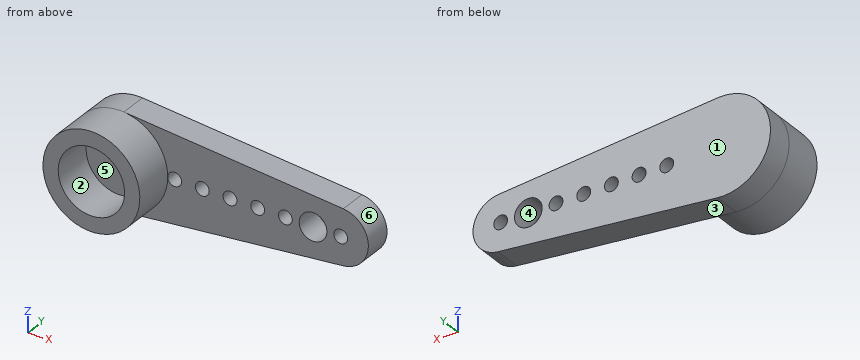
from build123d import *

# Parameters (mm, degrees)
SKETCH1_R           = 3.5
SKETCH1_R_2         = 2.4
BOSS_EXTRUDE1_DEPTH = 3
SKETCH2_R           = 1
SKETCH2_R_2         = 0.5
BOSS_EXTRUDE2_DEPTH = 2


with BuildPart() as part:
    # Sketch1 → Boss-Extrude1 (new body)
    with BuildSketch(Plane(origin=(0, 0, 0), x_dir=(1, 0, 0), z_dir=(0, 1, 0))):
        with Locations(Location((0, 0, 0), (0, 0, 270))):
            Circle(SKETCH1_R)
        with Locations(Location((0, 0, 0), (0, 0, 270))):
            Circle(SKETCH1_R_2, mode=Mode.SUBTRACT)
    extrude(amount=BOSS_EXTRUDE1_DEPTH)

    # Sketch2 → Boss-Extrude2 (add)
    with BuildSketch(Plane(origin=(0, 3, 0), x_dir=(1, 0, 0), z_dir=(0, 1, 0))):
        with BuildLine():
            Line((16.1875, 1.99119154), (0.328125, 3.484585195))
            ThreePointArc((0.328125, 3.484585195), (-3.5, 0), (0.328125, -3.484585195))
            Line((0.328125, -3.484585195), (16.1875, -1.99119154))
            ThreePointArc((16.1875, -1.99119154), (18, 0), (16.1875, 1.99119154))
        make_face()
        with Locations(Location((14, 0, 0), (0, 0, 270))):
            Circle(SKETCH2_R, mode=Mode.SUBTRACT)
        with Locations(Location((4, 0, 0), (0, 0, 180))):
            Circle(SKETCH2_R_2, mode=Mode.SUBTRACT)
        with Locations(Location((6, 0, 0), (0, 0, 270))):
            Circle(SKETCH2_R_2, mode=Mode.SUBTRACT)
        with Locations(Location((8, 0, 0), (0, 0, 270))):
            Circle(SKETCH2_R_2, mode=Mode.SUBTRACT)
        with Locations(Location((10, 0, 0), (0, 0, 270))):
            Circle(SKETCH2_R_2, mode=Mode.SUBTRACT)
        with Locations(Location((12, 0, 0), (0, 0, 270))):
            Circle(SKETCH2_R_2, mode=Mode.SUBTRACT)
        with Locations(Location((16, 0, 0), (0, 0, 270))):
            Circle(SKETCH2_R_2, mode=Mode.SUBTRACT)
    extrude(amount=BOSS_EXTRUDE2_DEPTH)


solid = part.part
Input: part model. Units: mm. Frame: model coordinates. Face numbers are marked on the shaded views. A direction names the side the tool comes from. Coordinates: 2 decimals unless noted, no trailing zeros. Loops run counter-clockwise (first coordinate to the right, second up) from the corner with the lowest first, then second, coordinate; pieces in that order, holes last.
Q1. Cut plane B-B (y = 3.65). Output: boundary loops of the cut face in (x, z).
Q2. Set-up query: the marked faces 5 and 6. Return all of +Z, -Z, +X, -X, +Y, -Y with unobstructed straight access to the full face (end or side cutting, diameter ignored); none if empty.
Q3. Cut plane A-A (x = 4). Output: boundary loops of the cut face in (y, z), then the cut area to 3 significant figures.
Q4. Material intervals for line 1 (X direction, y = 1.65, z = 0); line 2 (X direction, y = 1.9, z = -2); line 3 (Y direction, x = -1.5, z = 1), sorted ascending.
Q5. Cut plane C-C (x = 0). Output: boundary loops of the cut face in (y, z).
Q6. Draft query along Z for the marked faces 1, 2, 3 and 4. Return one class per face: +Z half, -Z half, draft (parallel to the pull), parting line (faces both ways), or undercut.
Q7. Cut plane D-D (y = 0.6). Output: boundary loops of the cut face in (x, z).
Q8. Contact query for flat-ended pins moving along their axis: pin 1 (1.8 mm diameter, centred on x = 14, z = 0, fed in from -Y); pin 2 (3 mm diameter, centred on y = 3, z = -2.5, fed in from +X); pin 3 (4 mm diameter, centred on x = 7.5, z = -2.5, fed in from -Y). Output: stop coordinate, or through.
Working result:
1. outline: (0.33, -3.48) - (16.19, -1.99) arc R2 ccw to (16.19, 1.99) - (0.33, 3.48) arc R3.5 ccw (long way) to start; hole circle Ø1 at (4, 0); hole circle Ø1 at (6, 0); hole circle Ø1 at (8, 0); hole circle Ø1 at (10, 0); hole circle Ø1 at (12, 0); hole circle Ø2 at (14, 0); hole circle Ø1 at (16, 0)
2. face 5: -Y
2. face 6: +X, +Y, -Y
3. outline: (3, -3.14) - (5, -3.14) - (5, -0.5) - (3, -0.5) - close; (3, 0.5) - (5, 0.5) - (5, 3.14) - (3, 3.14) - close
3. area: 10.6 mm2
4. line 1: x = -3.5 to -2.4, 2.4 to 3.5
4. line 2: x = -2.87 to -1.33, 1.33 to 2.87
4. line 3: y = 3 to 5
5. outline: (0, -3.5) - (5, -3.5) - (5, 3.5) - (0, 3.5) - (0, 2.4) - (3, 2.4) - (3, -2.4) - (0, -2.4) - close
6. face 1: draft
6. face 2: undercut
6. face 3: -Z half
6. face 4: undercut
7. outline: circle Ø7 at (0, 0); hole circle Ø4.8 at (0, 0)
8. pin 1: passes through
8. pin 2: stops at x = 17.73
8. pin 3: stops at y = 3
